```python
from build123d import *

# Parameters (mm, degrees)
SCHIZZO2_W                = 20
SCHIZZO2_H                = 10
SCHIZZO2_W_2              = 18
SCHIZZO2_H_2              = 8
ESTRUSIONE_SOTTILE1_DEPTH = 100
SCHIZZO3_R                = 3
TAGLIO_ESTRUSIONE1_DEPTH  = 101.995049384
RACCORDO6_R               = 1


with BuildPart() as part:
    # Schizzo2 → Estrusione-Sottile1 (new body)
    with BuildSketch(Plane(origin=(0, 0, 0), x_dir=(1, 0, 0), z_dir=(0, 1, 0))):
        Rectangle(SCHIZZO2_W, SCHIZZO2_H)
        Rectangle(SCHIZZO2_W_2, SCHIZZO2_H_2, mode=Mode.SUBTRACT)
    extrude(amount=-ESTRUSIONE_SOTTILE1_DEPTH)

    # Schizzo3 → Taglio-Estrusione1 (cut, through all)
    with BuildSketch(Plane.XY.offset(5)):
        with Locations((0, -5)):
            Circle(SCHIZZO3_R)
    extrude(amount=-TAGLIO_ESTRUSIONE1_DEPTH, mode=Mode.SUBTRACT)

    # Raccordo6
    raccordo6_edges = [part.edges().sort_by_distance(p)[0] for p in [
        (10, -50, 5),
        (-10, -50, 5),
        (-10, -50, -5),
        (10, -50, -5),
    ]]
    fillet(raccordo6_edges, radius=RACCORDO6_R)


solid = part.part
```
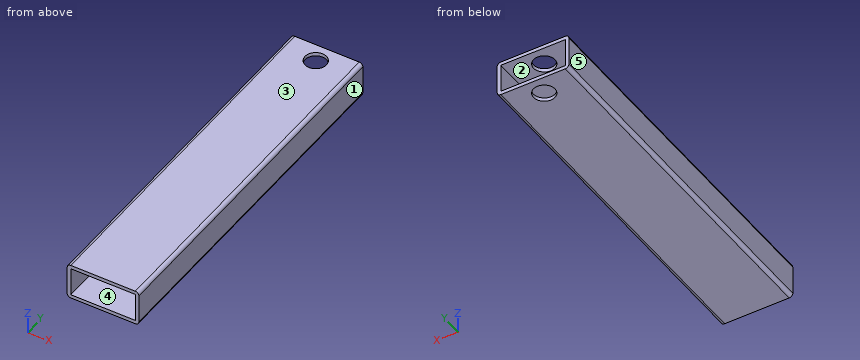
Verification items for the finished model (mm, model axes). Face numbers are marked on the shaded views. A direction names the side the tool comes from. Coordinates: 2 decimals unless noted, no trailing zeros. Loops run counter-clockwise (first coordinate to the right, second up) from the corner with the lowest first, then second, coordinate; pieces in that order, holes last. Notation, with made-up numbers: (39.25, 16.25) -> (49.25, 16.25) arc R16 cw to (49.25, 41.25) -> close; hole circle Ø2 at (-7, -37). An arc over 180 degrees is marked (long way). Answer in a Markdown table with one row per item.
1) Section check D-D (y = -5). Record the cut outline in (x, z).
The answers:
| item | result |
|---|---|
| outline | (-10, -4) arc R1 ccw to (-9, -5) -> (-3, -5) -> (-3, -4) -> (-9, -4) -> (-9, 4) -> (-3, 4) -> (-3, 5) -> (-9, 5) arc R1 ccw to (-10, 4) -> close; (3, -5) -> (9, -5) arc R1 ccw to (10, -4) -> (10, 4) arc R1 ccw to (9, 5) -> (3, 5) -> (3, 4) -> (9, 4) -> (9, -4) -> (3, -4) -> close |
2) Access from +Z, -Z, +X, -X, +Y, -Y to the whole of each face (thin tool, end or side, straight path). Record for the marked faces 4 and 5.
The answers:
| item | result |
|---|---|
| face 4 | +Y, -Y |
| face 5 | +Z, -Z, -X, +Y, -Y |
3) Section check A-A (x = 6.25). Record the cut outline in (y, z), and give its area (3 significant figures).
The answers:
| item | result |
|---|---|
| outline | (-100, -5) -> (0, -5) -> (0, -4) -> (-100, -4) -> close; (-100, 4) -> (0, 4) -> (0, 5) -> (-100, 5) -> close |
| area | 200 mm2 |
4) Scan lines: line 1 along Z through (x, y) = (3.5, -85); line 2 along Y through (x, z) = (0, 4.6); line 3 along Z through (x, y) = (9.25, -88). Record each from-to range of solid material in increasing order. Write a range as from..to.
The answers:
| item | result |
|---|---|
| line 1 | z = -5..-4, 4..5 |
| line 2 | y = -100..-8, -2..0 |
| line 3 | z = -4.97..4.97 |
5) Draft check along Z on the marked faces 1, 2 and 3. Enter one of: released by +Z, released by -Z, zero draft, split by the parting line, or undercut.
The answers:
| item | result |
|---|---|
| face 1 | zero draft |
| face 2 | undercut |
| face 3 | released by +Z |
6) Section check C-C (x = 0). Record the cut outline in (y, z), and give its area (3 significant figures).
The answers:
| item | result |
|---|---|
| outline | (-100, -5) -> (-8, -5) -> (-8, -4) -> (-100, -4) -> close; (-100, 4) -> (-8, 4) -> (-8, 5) -> (-100, 5) -> close; (-2, -5) -> (0, -5) -> (0, -4) -> (-2, -4) -> close; (-2, 4) -> (0, 4) -> (0, 5) -> (-2, 5) -> close |
| area | 188 mm2 |
7) Section check B-B (z = -1.25). Record the cut outline in (x, y), and give its area (3 significant figures).
The answers:
| item | result |
|---|---|
| outline | (-10, -100) -> (-9, -100) -> (-9, 0) -> (-10, 0) -> close; (9, -100) -> (10, -100) -> (10, 0) -> (9, 0) -> close |
| area | 200 mm2 |
